Build history of the part. All positions in model axes, mm. A direction names the side the tool comes from. Give positions to 0.01 mm unless a question says otherwise; leave off trailing zeros. Order: outer loops, then holes, each group sorted by start corner. A loop starts at its lowest first (then second) coordinate and runs counter-clockwise, first axis right, second up. Notation, with made-up numbers: (81.25, 89) - (137.25, 89) arc R36 cw to (137.25, 126) - close; hole circle Ø6 at (-9, -12.5). An arc over 180 degrees is marked (long way). Write each question's results on one line, items separated by ' | '. Start each with the question number.
1) Two-plate mould, pull along X, no slides. Class faces 3 (the face through (-2.5, 37, 15)), 4 (the face through (47, 38, 0)), 5 (the face through (98.5, 37, 15)): +X half, -X half, draft (parallel to the pull), parting line (faces both ways), or undercut.
2) Cut at B-B on x = 21.5. List the corners of the cut face in (y, z), plus the area to 3 significant figures.
3) Drill centre lines: line 1 along Y through (x, z) = (28.5, 27.5); line 2 along X through (y, z) = (3.5, 20.25); line 3 along Z through (x, y) = (48, 49.5). Where is each one in solid material? Low to high. Write a range as from..to.
4) Cut at C-C on y = 20. List the corners of the cut face in (x, z), plus the area to 3 significant figures.
5) Tool access for faces 1 (the face through (47, 77.5, 15)), 2 (the face through (47, -3.5, 15)): list every direction of +Z, -Z, +X, -X, +Y, -Y with a clear straight run to the whole face (end or side of a thin tool).
6) Cut at A-A on z = 13.75. List the corners of the cut face in (x, y).
from build123d import *

# Parameters (mm, degrees)
BOX002_W     = 110
BOX002_H     = 100
BOX002_DEPTH = 20
BOX001_W     = 100
BOX001_H     = 80
BOX001_DEPTH = 50
BOX_W        = 102
BOX_H        = 82
BOX_DEPTH    = 50
FILLET_R     = 0.25


with BuildPart() as cube002:
    # Box002 → Box002 (new body)
    with BuildSketch(Plane(origin=(-10, -10, 30), x_dir=(1, 0, 0), z_dir=(0, 0, 1))):
        with Locations((55, 50)):
            Rectangle(BOX002_W, BOX002_H)
    extrude(amount=BOX002_DEPTH)


with BuildPart() as cube001:
    # Box001 → Box001 (new body)
    with BuildSketch(Plane(origin=(1, 1, 1), x_dir=(1, 0, 0), z_dir=(0, 0, 1))):
        with Locations((50, 40)):
            Rectangle(BOX001_W, BOX001_H)
    extrude(amount=BOX001_DEPTH)


with BuildPart() as box:
    # Box → Box (new body)
    with BuildSketch(Plane.XY):
        with Locations((51, 41)):
            Rectangle(BOX_W, BOX_H)
    extrude(amount=BOX_DEPTH)

    # Cut: cut Cube001
    add(cube001.part, mode=Mode.SUBTRACT)

    # Fillet
    fillet_edges = [box.edges().sort_by_distance(p)[0] for p in [
        (0, 0, 25),
        (0, 41, 50),
        (0, 82, 25),
        (0, 41, 0),
        (51, 0, 0),
        (102, 0, 25),
        (51, 0, 50),
        (51, 82, 50),
        (102, 41, 50),
        (51, 1, 50),
        (101, 41, 50),
        (51, 81, 50),
        (1, 41, 50),
        (51, 82, 0),
        (102, 82, 25),
        (102, 41, 0),
        (101, 1, 25.5),
        (1, 1, 25.5),
        (51, 1, 1),
        (101, 81, 25.5),
        (101, 41, 1),
        (1, 81, 25.5),
        (51, 81, 1),
        (1, 41, 1),
    ]]
    fillet(fillet_edges, radius=FILLET_R)


with BuildPart() as box_1:
    # Fillet placement: moved
    add(box.part.moved(Location((-3.5, -3.5, 0))))

    # Cut005: cut Cube002
    add(cube002.part, mode=Mode.SUBTRACT)


solid = box_1.part
Results:
1) face 3: undercut | face 4: draft | face 5: +X half
2) outline: (-3.5, 0.25) arc R0.25 ccw to (-3.25, 0) - (78.25, 0) arc R0.25 ccw to (78.5, 0.25) - (78.5, 30) - (77.5, 30) - (77.5, 1.25) arc R0.25 cw to (77.25, 1) - (-2.25, 1) arc R0.25 cw to (-2.5, 1.25) - (-2.5, 30) - (-3.5, 30) - close | area: 140 mm^2
3) line 1: -3.5..-2.5, 77.5..78.5 | line 2: -3.5..-2.5, 97.5..98.5 | line 3: 0..1
4) outline: (-3.5, 0.25) arc R0.25 ccw to (-3.25, 0) - (98.25, 0) arc R0.25 ccw to (98.5, 0.25) - (98.5, 30) - (97.5, 30) - (97.5, 1.25) arc R0.25 cw to (97.25, 1) - (-2.25, 1) arc R0.25 cw to (-2.5, 1.25) - (-2.5, 30) - (-3.5, 30) - close | area: 160 mm^2
5) face 1: +Z | face 2: +Z, -Z, +X, -X, -Y
6) outline: (-3.5, -3.25) arc R0.25 ccw to (-3.25, -3.5) - (98.25, -3.5) arc R0.25 ccw to (98.5, -3.25) - (98.5, 78.25) arc R0.25 ccw to (98.25, 78.5) - (-3.25, 78.5) arc R0.25 ccw to (-3.5, 78.25) - close; hole (-2.5, -2.25) arc R0.25 ccw to (-2.25, -2.5) - (97.25, -2.5) arc R0.25 ccw to (97.5, -2.25) - (97.5, 77.25) arc R0.25 ccw to (97.25, 77.5) - (-2.25, 77.5) arc R0.25 ccw to (-2.5, 77.25) - close
